```python
from build123d import *

# Parameters (mm, degrees)
PAD_DEPTH          = 120
POCKET_DEPTH       = 380
POLARPATTERN_COUNT = 4
POCKET001_DEPTH    = 380


with BuildPart() as part:
    # Sketch → Pad (new body)
    with BuildSketch(Plane.XZ):
        with BuildLine():
            Line((-9, 10), (9, 10))
            ThreePointArc((10, 9), (9.707107, 9.707107), (9, 10))
            Line((10, 9), (10, -9))
            ThreePointArc((9, -10), (9.707107, -9.707107), (10, -9))
            Line((9, -10), (-9, -10))
            ThreePointArc((-10, -9), (-9.707107, -9.707107), (-9, -10))
            Line((-10, -9), (-10, 9))
            ThreePointArc((-9, 10), (-9.707107, 9.707107), (-10, 9))
        make_face()
    extrude(amount=PAD_DEPTH)

    # Sketch001 (on Face10 of Pad) → Pocket (cut)
    with BuildSketch(Plane.XZ.offset(120)):
        Polygon((-3.4, 10), (-3.4, 9.6), (-3, 9.6), (-3, 8.5), (-6, 8.5), (-6, 7), (-3.35, 4.7), (-0.65, 4.7), (0, 4.3), (0.65, 4.7), (3.35, 4.7), (6, 7), (6, 8.5), (3, 8.5), (3, 9.6), (3.4, 9.6), (3.4, 10), align=None)
    pocket = extrude(amount=-POCKET_DEPTH, mode=Mode.SUBTRACT)

    # PolarPattern: Pocket ×4 about axis
    polarpattern_axis = Axis((0, -120, 0), (0, -1, 0))
    for i in range(1, POLARPATTERN_COUNT):
        add(pocket.rotate(polarpattern_axis, i * 360 / POLARPATTERN_COUNT), mode=Mode.SUBTRACT)

    # Sketch002 (on Face4 of PolarPattern) → Pocket001 (cut)
    with BuildSketch(Plane.XZ.offset(120)):
        with BuildLine():
            ThreePointArc((1.340499, 2.401159), (0, 2.75), (-1.340499, 2.401159))
            Line((-1.944544, 3.005204), (-1.340499, 2.401159))
            Line((-3.005204, 1.944544), (-1.944544, 3.005204))
            Line((-2.401159, 1.340499), (-3.005204, 1.944544))
            ThreePointArc((-2.401159, 1.340499), (-2.75, 0), (-2.401159, -1.340499))
            Line((-3.005204, -1.944544), (-2.401159, -1.340499))
            Line((-1.944544, -3.005204), (-3.005204, -1.944544))
            Line((-1.340499, -2.401159), (-1.944544, -3.005204))
            ThreePointArc((-1.340499, -2.401159), (0, -2.75), (1.340499, -2.401159))
            Line((1.944544, -3.005204), (1.340499, -2.401159))
            Line((3.005204, -1.944544), (1.944544, -3.005204))
            Line((2.401159, -1.340499), (3.005204, -1.944544))
            ThreePointArc((2.401159, -1.340499), (2.75, 0), (2.401159, 1.340499))
            Line((2.401159, 1.340499), (3.005204, 1.944544))
            Line((3.005204, 1.944544), (1.944544, 3.005204))
            Line((1.944544, 3.005204), (1.340499, 2.401159))
        make_face()
    extrude(amount=-POCKET001_DEPTH, mode=Mode.SUBTRACT)


solid = part.part
```
Could you check a few things on this model? Use its own coordinates, in mm. A direction names the side the tool comes from. Round coordinates to 2 decimals unless told otherwise and drop trailing zeros. Write item = value, one per line.
1. I need wall thicknesses on probe 1 along X at (y, z) = (-77, -8.75); probe 2 along Z at (x, y) = (5.25, -55); probe 3 along X at (y, z) = (-105, 5.75). Which ranges of each line are inside material? Lowest first, please.
Results below:
probe_1 = -10 to -3, 3 to 10
probe_2 = -10 to -8.5, -6.35 to -3.98, 3.98 to 6.35, 8.5 to 10
probe_3 = -10 to -8.5, -6.78 to -4.56, 4.56 to 6.78, 8.5 to 10
2. Which directions (+Z, -Z, +X, -X, +Y, -Y) give clear straight access to the entire face, cutting with the end or side of a thin tool? Please do faces 1 (the face through (4.656, -60.84, 5.834)), 2 (the face through (-4, -120, 0)).
Results below:
face_1 = +Y, -Y
face_2 = +Z, -Z, +X, -X, -Y
3. Thinking about a two-plate mould opening in Z: for faces 3 (the face through (-6, -59, 10)), 4 (the face through (-6, -59, -10)), 5 (the face through (8.5, -61, 4)), which applies, +Z half, -Z half, draft (parallel to the pull), parting line (faces both ways), or undercut?
Results below:
face_3 = +Z half
face_4 = -Z half
face_5 = undercut
4. Will these pins go through, and if not, where does the flat tip stop? P1, Ø1.4, axis at y = -58, z = 1.5, coming from the +X side; P2, Ø2, axis at x = 0.5, y = -100.5, coming from the +Z side.
Results below:
P1 = 4.7
P2 = 4.7
